The model under review builds one solid part; all positions refer to its coordinate system, in mm. A direction names the side the tool comes from. Give positions to 0.01 mm unless a question says otherwise; leave off trailing zeros. Loops run counter-clockwise (first coordinate to the right, second up) from the corner with the lowest first, then second, coordinate; pieces in that order, holes last. Notation, with made-up numbers: M 32.25,2 L 72.25,2 A10 cw 72.25,17 Z; hole C 23,-21 d2. An arc over 180 degrees is marked long. Return JSON: item names as keys, results as strings.
```python
from build123d import *

# Parameters (mm, degrees)
F0_W     = 25.4
F0_H     = 25.4
F1_DEPTH = 24.638
F2_W     = 50.8
F2_H     = 50.8
F3_DEPTH = 25.4


with BuildPart() as f1:
    # F0 (on Front) → F1 (new body)
    with BuildSketch(Plane.XZ):
        with Locations((-43.39072, 21.789327)):
            Rectangle(F0_W, F0_H)
    extrude(amount=F1_DEPTH)

    # F2 (on Top) → F3 (join)
    with BuildSketch(Plane.XY):
        with Locations((-43.128742, -25.4)):
            Rectangle(F2_W, F2_H)
    extrude(amount=F3_DEPTH)


solid = f1.part
```
1) Consider section A-A on y = -7. Write out the cut boundary in (x, z).
From the geometry:
{"outline": "M -68.53,0 L -17.73,0 L -17.73,25.4 L -30.69,25.4 L -30.69,34.49 L -56.09,34.49 L -56.09,25.4 L -68.53,25.4 Z"}
2) Consider section D-D on x = -27.5. Write out the cut boundary in (y, z), then the cut area to 3 significant figures.
From the geometry:
{"outline": "M -50.8,0 L 0,0 L 0,25.4 L -50.8,25.4 Z", "area": "1,290 mm²"}
3) Consider section C-C on y = -37. Write out the cut boundary in (x, z).
From the geometry:
{"outline": "M -68.53,0 L -17.73,0 L -17.73,25.4 L -68.53,25.4 Z"}
4) Wall thickness on L1, parallel to Z at x = -31.5, y = -43; L2, parallel to X at y = -5.5, z = 29; L3, parallel to Y at x = -56, z = 27: over which ranges is each line inside the solid? List them lowest first. Write a range as from..to.
From the geometry:
{"L1": "0..25.4", "L2": "-56.09..-30.69", "L3": "-24.64..0"}
5) Insertion check: pin 1 (1 mm diameter, centred on x = -54, y = -19.5, fed in from -Z); pin 2 (10 mm diameter, centred on y = -13.5, z = 31.5, fed in from -X); pin 3 (4.5 mm diameter, centred on y = -12, z = 28, fed in from +X); pin 4 (7.5 mm diameter, centred on x = -46, z = 31, fed in from -Y). Each pin has a flat end and moves straight along its axis. Give the tip position at first contact, or say it passes through.
From the geometry:
{"pin 1": "z = 0", "pin 2": "x = -56.09", "pin 3": "x = -30.69", "pin 4": "y = -24.64"}
6) Tool access review of faces 1 (the face through (-56.091, -12, 30)), 2 (the face through (-30.691, -12, 30)), 3 (the face through (-44, -24.638, 30)): name each direction out of +Z, -Z, +X, -X, +Y, -Y from which nothing blocks a thin tool from reaching the whole face with its end or side.
From the geometry:
{"face 1": "+Z, -X, +Y, -Y", "face 2": "+Z, +X, +Y, -Y", "face 3": "+Z, +X, -X, -Y"}
7) Consider section B-B on x = -53. Write out the cut boundary in (y, z), then the cut area to 3 significant figures.
From the geometry:
{"outline": "M -50.8,0 L 0,0 L 0,34.49 L -24.64,34.49 L -24.64,25.4 L -50.8,25.4 Z", "area": "1,510 mm²"}
